Verification items for the finished model (mm, model axes). A direction names the side the tool comes from. Round coordinates to 2 decimals unless told otherwise and drop trailing zeros. Write each loop counter-clockwise with the first axis right and the second up, starting at its lowest first coordinate (ties: lowest second). Pieces come first, ordered by that corner, then holes. Notation, with made-up numbers: (-38, -36.75) - (-11, -36.75) arc R17 cw to (-11, -18.75) - close; hole circle Ø11 at (86, -2). An arc over 180 degrees is marked (long way). Write each question's results on one line, items separated by ' | '.
```python
from build123d import *

# Parameters (mm, degrees)
SKETCH1_R           = 1.5875
BOSS_EXTRUDE1_DEPTH = 2.54
BOSS_EXTRUDE2_DEPTH = 8.255
SKETCH3_W           = 64.77
SKETCH3_H           = 7.1
CUT_EXTRUDE1_DEPTH  = 0.635
SKETCH9_R           = 1.5875
CUT_EXTRUDE4_DEPTH  = 89.512075769
SKETCH4_R           = 1.143
CUT_EXTRUDE2_DEPTH  = 11.43
BOSS_EXTRUDE5_DEPTH = 8.255
SKETCH28_R          = 1.5875
CUT_EXTRUDE12_DEPTH = 7.62
SKETCH29_R          = 1.5875
CUT_EXTRUDE13_DEPTH = 10.16
CUT_EXTRUDE14_START = -12.7
SKETCH30_R          = 1.5875
CUT_EXTRUDE14_DEPTH = 12.7
SKETCH31_R          = 1.5875
CUT_EXTRUDE15_DEPTH = 12.7
CUT_EXTRUDE16_START = -12.7
SKETCH32_R          = 1.5875
CUT_EXTRUDE16_DEPTH = 12.7
BOSS_EXTRUDE6_DEPTH = 2.54
CUT_EXTRUDE17_DEPTH = 89.512075921


with BuildPart() as part:
    # Sketch1 → Boss-Extrude1 (new body)
    with BuildSketch(Plane.XY):
        with BuildLine():
            Line((-71.572584947, 25.4), (-65.222584947, 25.4))
            Line((-65.222584947, 25.4), (-65.222584947, 22.86))
            ThreePointArc((-65.222584947, 22.86), (-63.362713008, 18.369871939), (-58.872584947, 16.51))
            Line((-58.872584947, 16.51), (44.196, 16.51))
            ThreePointArc((44.196, 16.51), (48.686128061, 18.369871939), (50.546, 22.86))
            Line((50.546, 22.86), (50.546, 44.45))
            Line((50.546, 44.45), (61.579155694, 44.45))
            ThreePointArc((61.579155694, 44.45), (75.946, 0), (61.579155694, -44.45))
            Line((61.579155694, -44.45), (50.546, -44.45))
            Line((50.546, -44.45), (50.546, -22.86))
            ThreePointArc((50.546, -22.86), (48.686128061, -18.369871939), (44.196, -16.51))
            Line((44.196, -16.51), (-58.872584947, -16.51))
            ThreePointArc((-58.872584947, -16.51), (-63.362713008, -18.369871939), (-65.222584947, -22.86))
            Line((-65.222584947, -22.86), (-65.222584947, -25.4))
            Line((-65.222584947, -25.4), (-71.572584947, -25.4))
            ThreePointArc((-71.572584947, -25.4), (-75.946, 0), (-71.572584947, 25.4))
        make_face()
        with Locations((-22.6695, 8.128)):
            Circle(SKETCH1_R, mode=Mode.SUBTRACT)
        with Locations((-22.6695, -8.128)):
            Circle(SKETCH1_R, mode=Mode.SUBTRACT)
    extrude(amount=BOSS_EXTRUDE1_DEPTH)

    # Sketch2 → Boss-Extrude2 (add)
    with BuildSketch(Plane.XY.offset(2.54)):
        with BuildLine():
            Line((61.865268471, 17.78), (60.095110466, 38.1))
            ThreePointArc((60.095110466, 38.1), (59.464196764, 40.158289632), (58.047089349, 41.778911391))
            Line((58.047089349, 41.778911391), (57.900800643, 44.704))
            Line((57.900800643, 44.704), (61.395010384, 44.704))
            ThreePointArc((61.395010384, 44.704), (69.822038137, 29.877715884), (74.728381149, 13.544887112))
            Line((74.728381149, 13.544887112), (60.759450402, 13.544887112))
            Line((60.759450402, 13.544887112), (60.759450402, 15.094127876))
            ThreePointArc((60.759450402, 15.094127876), (61.639191639, 16.302501703), (61.865268471, 17.78))
        make_face()
        with BuildLine():
            Line((58.651639318, 17.500047669), (56.881481313, 37.820047669))
            Line((56.881481313, 37.820047669), (50.546, 37.820047669))
            Line((50.546, 37.820047669), (50.546, 16.566735288))
            Line((50.546, 16.566735288), (57.366094516, 16.566735288))
            ThreePointArc((57.366094516, 16.566735288), (58.160401987, 16.824667019), (58.651639318, 17.500047669))
        make_face()
        with BuildLine():
            Line((60.759450402, -13.544887112), (74.728381149, -13.544887112))
            ThreePointArc((74.728381149, -13.544887112), (69.822038137, -29.877715884), (61.395010384, -44.704))
            Line((61.395010384, -44.704), (57.900800643, -44.704))
            Line((57.900800643, -44.704), (58.047089349, -41.778911391))
            ThreePointArc((58.047089349, -41.778911391), (59.464196764, -40.158289632), (60.095110466, -38.1))
            Line((60.095110466, -38.1), (61.865268471, -17.78))
            ThreePointArc((61.865268471, -17.78), (61.639191639, -16.302501703), (60.759450402, -15.094127876))
            Line((60.759450402, -15.094127876), (60.759450402, -13.544887112))
        make_face()
        with BuildLine():
            Line((50.546, -16.566735288), (57.366094516, -16.566735288))
            ThreePointArc((57.366094516, -16.566735288), (58.160401987, -16.824667019), (58.651639318, -17.500047669))
            Line((58.651639318, -17.500047669), (56.881481313, -37.820047669))
            Line((56.881481313, -37.820047669), (50.546, -37.820047669))
            Line((50.546, -37.820047669), (50.546, -16.566735288))
        make_face()
    extrude(amount=BOSS_EXTRUDE2_DEPTH)

    # Sketch3 → Cut-Extrude1 (cut)
    with BuildSketch(Plane.XY.offset(2.54)):
        with Locations((44.577, 0)):
            Rectangle(SKETCH3_W, SKETCH3_H)
    extrude(amount=-CUT_EXTRUDE1_DEPTH, mode=Mode.SUBTRACT)

    # Sketch9 → Cut-Extrude4 (cut, through all)
    with BuildSketch(Plane.XY.offset(2.54)):
        with Locations((72.560984492, -7.239)):
            Circle(SKETCH9_R)
        with Locations((72.560984492, 7.239)):
            Circle(SKETCH9_R)
    extrude(amount=-CUT_EXTRUDE4_DEPTH, mode=Mode.SUBTRACT)

    # Sketch4 → Cut-Extrude2 (cut)
    with BuildSketch(Plane.XY.offset(1.905)):
        with Locations((19.812, 0)):
            Circle(SKETCH4_R)
        with Locations((34.798, 0)):
            Circle(SKETCH4_R)
        with Locations((49.784, 0)):
            Circle(SKETCH4_R)
        with Locations((64.77, 0)):
            Circle(SKETCH4_R)
    extrude(amount=-CUT_EXTRUDE2_DEPTH, mode=Mode.SUBTRACT)

    # Sketch19 → Boss-Extrude5 (add)
    with BuildSketch(Plane.XY.offset(2.54)):
        with BuildLine():
            Line((-71.572584947, -25.4), (-65.222584947, -25.4))
            Line((-65.222584947, -25.4), (-65.222584947, 25.4))
            Line((-65.222584947, 25.4), (-71.572584947, 25.4))
            ThreePointArc((-71.572584947, 25.4), (-75.946, 0), (-71.572584947, -25.4))
        make_face()
    extrude(amount=BOSS_EXTRUDE5_DEPTH)

    # Sketch28 → Cut-Extrude12 (cut)
    with BuildSketch(Plane(origin=(65.771165316, 37.973, 0), x_dir=(0, 0, -1), z_dir=(0.8660254037844379, 0.5000000000000011, 0))):
        with Locations(Location((-6.053310192, 0, 0), (0, 0, 90))):
            Circle(SKETCH28_R)
    cut_extrude12 = extrude(amount=-CUT_EXTRUDE12_DEPTH, mode=Mode.SUBTRACT)

    # Sketch29 → Cut-Extrude13 (cut)
    with BuildSketch(Plane(origin=(73.358202803, 19.656271199, 0), x_dir=(0, 0, -1), z_dir=(0.9659258262890682, 0.25881904510252135, 0))):
        with Locations(Location((-6.096, 0, 0), (0, 0, 90))):
            Circle(SKETCH29_R)
    cut_extrude13 = extrude(amount=-CUT_EXTRUDE13_DEPTH, mode=Mode.SUBTRACT)

    # Mirror3: Cut-Extrude12, Cut-Extrude13 across plane
    add(cut_extrude12.mirror(Plane.ZX), mode=Mode.SUBTRACT)
    add(cut_extrude13.mirror(Plane.ZX), mode=Mode.SUBTRACT)

    # Sketch30 → Cut-Extrude14 (cut)
    with BuildSketch(Plane(origin=(-73.358202803, 19.656271199, 0), x_dir=(0, 0, 1), z_dir=(-0.9659258262890681, 0.2588190451025213, 0)).offset(CUT_EXTRUDE14_START)):
        with Locations(Location((6.096, 0, 0), (0, 0, 90))):
            Circle(SKETCH30_R)
    extrude(amount=CUT_EXTRUDE14_DEPTH, mode=Mode.SUBTRACT)

    # Sketch31 → Cut-Extrude15 (cut)
    with BuildSketch(Plane.ZY.offset(75.946)):
        with Locations((6.096, 0)):
            Circle(SKETCH31_R)
    extrude(amount=-CUT_EXTRUDE15_DEPTH, mode=Mode.SUBTRACT)

    # Sketch32 → Cut-Extrude16 (cut)
    with BuildSketch(Plane(origin=(-73.358202803, -19.656271199, 0), x_dir=(0, 0, 1), z_dir=(-0.9659258262890681, -0.2588190451025213, 0)).offset(CUT_EXTRUDE16_START)):
        with Locations(Location((6.096, 0, 0), (0, 0, 90))):
            Circle(SKETCH32_R)
    extrude(amount=CUT_EXTRUDE16_DEPTH, mode=Mode.SUBTRACT)

    # Sketch33 → Boss-Extrude6 (add)
    with BuildSketch(Plane.XY.offset(2.54)):
        with BuildLine():
            Line((12.137284041, 16.51), (-58.872584947, 16.51))
            ThreePointArc((-58.872584947, 16.51), (-63.362713008, 18.369871939), (-65.222584947, 22.86))
            Line((-65.222584947, 22.86), (-65.222584947, 7.62))
            ThreePointArc((-65.222584947, 7.62), (-63.362713008, 12.110128061), (-58.872584947, 13.97))
            Line((-58.872584947, 13.97), (12.137284041, 13.97))
            Line((12.137284041, 13.97), (12.137284041, 16.51))
        make_face()
        with BuildLine():
            Line((12.137284041, -13.97), (12.137284041, -16.51))
            Line((12.137284041, -16.51), (-58.872584947, -16.51))
            ThreePointArc((-58.872584947, -16.51), (-63.362713008, -18.369871939), (-65.222584947, -22.86))
            Line((-65.222584947, -22.86), (-65.222584947, -7.62))
            ThreePointArc((-65.222584947, -7.62), (-63.362713008, -12.110128061), (-58.872584947, -13.97))
            Line((-58.872584947, -13.97), (12.137284041, -13.97))
        make_face()
    extrude(amount=BOSS_EXTRUDE6_DEPTH)

    # Sketch34 → Cut-Extrude17 (cut, through all)
    with BuildSketch(Plane.XY.offset(2.54)):
        with BuildLine():
            Line((-54.541546126, -10.16), (-34.358453874, -10.16))
            ThreePointArc((-34.358453874, -10.16), (-30.268934421, -8.466065579), (-28.575, -4.376546126))
            Line((-28.575, -4.376546126), (-28.575, 4.376546126))
            ThreePointArc((-28.575, 4.376546126), (-30.268934421, 8.466065579), (-34.358453874, 10.16))
            Line((-34.358453874, 10.16), (-54.541546126, 10.16))
            ThreePointArc((-54.541546126, 10.16), (-58.631065579, 8.466065579), (-60.325, 4.376546126))
            Line((-60.325, 4.376546126), (-60.325, -4.376546126))
            ThreePointArc((-60.325, -4.376546126), (-58.631065579, -8.466065579), (-54.541546126, -10.16))
        make_face()
        with BuildLine():
            Line((-9.525, 10.16), (0.635, 10.16))
            ThreePointArc((0.635, 10.16), (5.125128061, 8.300128061), (6.985, 3.81))
            Line((6.985, 3.81), (6.985, -3.81))
            ThreePointArc((6.985, -3.81), (5.125128061, -8.300128061), (0.635, -10.16))
            Line((0.635, -10.16), (-9.525, -10.16))
            ThreePointArc((-9.525, -10.16), (-14.015128061, -8.300128061), (-15.875, -3.81))
            Line((-15.875, -3.81), (-15.875, 3.81))
            ThreePointArc((-15.875, 3.81), (-14.015128061, 8.300128061), (-9.525, 10.16))
        make_face()
    extrude(amount=-CUT_EXTRUDE17_DEPTH, mode=Mode.SUBTRACT)


solid = part.part
```
(1) Set-up check for faces 4 (the flat face through (54, 16.567, 7)), 5 (the cylindrical face through (-63.31, 18.32, 2.5)), 6 (the flat face through (-30, 16, 5.08)), 7 (the flat face through (57.973, -43.262, 6.61)), 8 (the cylindrical face through (-30.314, -8.511, 1.288)): record each of +Z, -Z, +X, -X, +Y, -Y from which the full face is reachable in a straight line by a thin tool's end or side.
Answer:
face 4: +Z | face 5: +Z, -Z, +Y | face 6: +Z, +Y, -Y | face 7: +Z, -X | face 8: +Z, -Z
(2) Mould release check, pull along Z, two halves, no side actions. Record for faces 1 (the flat face through (55, -27, 10.795)), 2 (the flat face through (63.55, 17.01, 6.12)), 3 (the cylindrical face through (5.174, -8.25, 1.288)): released by +Z, released by -Z, zero draft, split by the parting line, or undercut.
Answer:
face 1: released by +Z | face 2: undercut | face 3: zero draft
(3) Section check A-A (x = -47). Record the cut outline in (y, z).
Answer:
outline: (-16.51, 0) - (-10.16, 0) - (-10.16, 2.54) - (-13.97, 2.54) - (-13.97, 5.08) - (-16.51, 5.08) - close; (10.16, 0) - (16.51, 0) - (16.51, 5.08) - (13.97, 5.08) - (13.97, 2.54) - (10.16, 2.54) - close
(4) Thickness scan on L1, parallel to Y at x = 51, z = 5; L2, parallel to X at y = -17.5, z = 10.5; L3, parallel to Y at x = -55, z = 3.5. Record the ranges inside material, lowest first.
Answer:
L1: -37.82 to -16.57, 16.57 to 37.82 | L2: -73.9 to -65.22, 50.55 to 58.65, 61.88 to 73.9 | L3: -16.51 to -13.97, 13.97 to 16.51
(5) Go/stop test with flat-tipped pins: pin 1 Ø4 at (x, y) = (-22.67, -8.13) entering from +Z; pin 2 Ø0.8 at (x, z) = (-37, 4) entering from -Y; pin 3 Ø2 at (y, z) = (-15.5, 8.5) entering from -X. Record where each tip stops, or that it passes through.
Answer:
pin 1: z = 2.54 | pin 2: y = -16.51 | pin 3: x = -74.55
